Can you work these out from the model? Positions are in its coordinate system, mm. A direction names the side the tool comes from. Coordinates: 2 decimals unless noted, no trailing zeros. Order: outer loops, then holes, each group sorted by start corner. A loop starts at its lowest first (then second) coordinate and runs counter-clockwise, first axis right, second up. Notation, with made-up numbers: (3.25, 71) - (8.25, 71) arc R29 cw to (8.25, 104) - close; hole circle Ø2 at (83, 62.25). An arc over 180 degrees is marked (long way). Return JSON: item names as keys, results as strings. Group by question number.
1) Imagine slicing it at A-A (y = -18.5). Write out the boundary of the cut face in (x, z).
2) For pin 1 Ø1.9 at (x, z) = (-18, 2.5) entering from -Y; pin 2 Ø1.5 at (y, z) = (16, 4) entering from -X; pin 3 Ø3 at (y, z) = (40.5, 3.5) entering from +X, each with a flat end and sliding along its axis, tell me the tip position at first contact or that it passes through.
3) Imagine slicing it at C-C (z = 1.75). Give the number of separate pieces and of enclosed holes in the cut face, and give its area (3 significant figures).
4) If I drill on line 1 along Y through (x, z) = (-101, 3.5); line 2 along X through (y, z) = (25, 4.25), over which ranges is the centre line in solid material (lowest first)?
5) If we mould it in two halves opening along X, with no side actions, what happens to faces 6 (the face through (31, 6.35, 3)), 7 (the face through (-57.15, 66, 3)), 8 (the face through (-50.8, 25, 3))? For each: pulls with the +X half, pulls with the -X half, needs draft (parallel to the pull), parting line crosses it, or undercut.
6) Imagine slicing it at B-B (x = 17). Write out the boundary of the cut face in (y, z), and give its area (3 significant figures).
7) Which directions (+Z, -Z, +X, -X, +Y, -Y) give clear straight access to the entire face, cutting with the end or side of a thin tool? Please do faces 1 (the face through (-26, 50.8, 3)), 2 (the face through (-83, 50.8, 3)), 3 (the face through (31, 0, 3)), 4 (the face through (31, 50.8, 3)), 5 (the face through (0, -29, 3)).
```python
from build123d import *

# Parameters (mm, degrees)
F0_W     = 6.35
F0_H     = 31.75
F0_W_2   = 50.8
F0_H_2   = 6.35
F0_H_3   = 38.1
F0_H_4   = 76.2
F1_DEPTH = 6.35
F3_DEPTH = 63.5


with BuildPart() as f1:
    # F0 (on Top) → F1 (new body)
    with BuildSketch(Plane.XY):
        Polygon((-50.8, 82.55), (0, 82.55), (6.35, 82.55), (57.15, 82.55), (57.15, 88.9), (-107.95, 88.9), (-107.95, 82.55), (-57.15, 82.55), align=None)
        with Locations((-53.975, 66.675)):
            Rectangle(F0_W, F0_H)
        with Locations((3.175, 66.675)):
            Rectangle(F0_W, F0_H)
        with Locations((31.75, 47.625)):
            Rectangle(F0_W_2, F0_H_2)
        with Locations((3.175, 47.625)):
            Rectangle(F0_W, F0_H_2)
        with Locations((-25.4, 47.625)):
            Rectangle(F0_W_2, F0_H_2)
        with Locations((-82.55, 47.625)):
            Rectangle(F0_W_2, F0_H_2)
        with Locations((-53.975, 47.625)):
            Rectangle(F0_W, F0_H_2)
        with Locations((-53.975, 25.4)):
            Rectangle(F0_W, F0_H_3)
        with Locations((3.175, 25.4)):
            Rectangle(F0_W, F0_H_3)
        with Locations((3.175, -38.1)):
            Rectangle(F0_W, F0_H_4)
        with Locations((3.175, 3.175)):
            Rectangle(F0_W, F0_H_2)
        with Locations((31.75, 3.175)):
            Rectangle(F0_W_2, F0_H_2)
        with Locations((-25.4, 3.175)):
            Rectangle(F0_W_2, F0_H_2)
        with Locations((-53.975, 3.175)):
            Rectangle(F0_W, F0_H_2)
        with Locations((-53.975, -38.1)):
            Rectangle(F0_W, F0_H_4)
        with Locations((-82.55, 3.175)):
            Rectangle(F0_W_2, F0_H_2)
    extrude(amount=F1_DEPTH)

    # F2 (on face) → F3 (cut, through all)
    with BuildSketch(Plane(origin=(-57.15, 0, 0), x_dir=(0, -1, 0), z_dir=(-1, 0, 0))):
        Polygon((53.4593649209, 6.35), (76.2, 0), (76.2, 6.35), align=None)
    extrude(amount=-F3_DEPTH, mode=Mode.SUBTRACT)


solid = f1.part
```
Calculated:
{
 "1": {"outline": "(-57.15, 0) - (-50.8, 0) - (-50.8, 6.35) - (-57.15, 6.35) - close; (0, 0) - (6.35, 0) - (6.35, 6.35) - (0, 6.35) - close"},
 "2": {"pin 1": "y = 0", "pin 2": "x = -57.15", "pin 3": "x = 6.35"},
 "3": {"separate pieces": "1", "enclosed holes": "2", "area": "4,920 mm2"},
 "4": {"line 1": "0 to 6.35, 44.45 to 50.8, 82.55 to 88.9", "line 2": "-57.15 to -50.8, 0 to 6.35"},
 "5": {"face 6": "needs draft", "face 7": "pulls with the -X half", "face 8": "undercut"},
 "6": {"outline": "(0, 0) - (6.35, 0) - (6.35, 6.35) - (0, 6.35) - close; (44.45, 0) - (50.8, 0) - (50.8, 6.35) - (44.45, 6.35) - close; (82.55, 0) - (88.9, 0) - (88.9, 6.35) - (82.55, 6.35) - close", "area": "121 mm2"},
 "7": {"face 1": "+Z, -Z", "face 2": "+Z, -Z, -X", "face 3": "+Z, -Z, +X, -Y", "face 4": "+Z, -Z, +X", "face 5": "+Z, -Z, -Y"}
}
